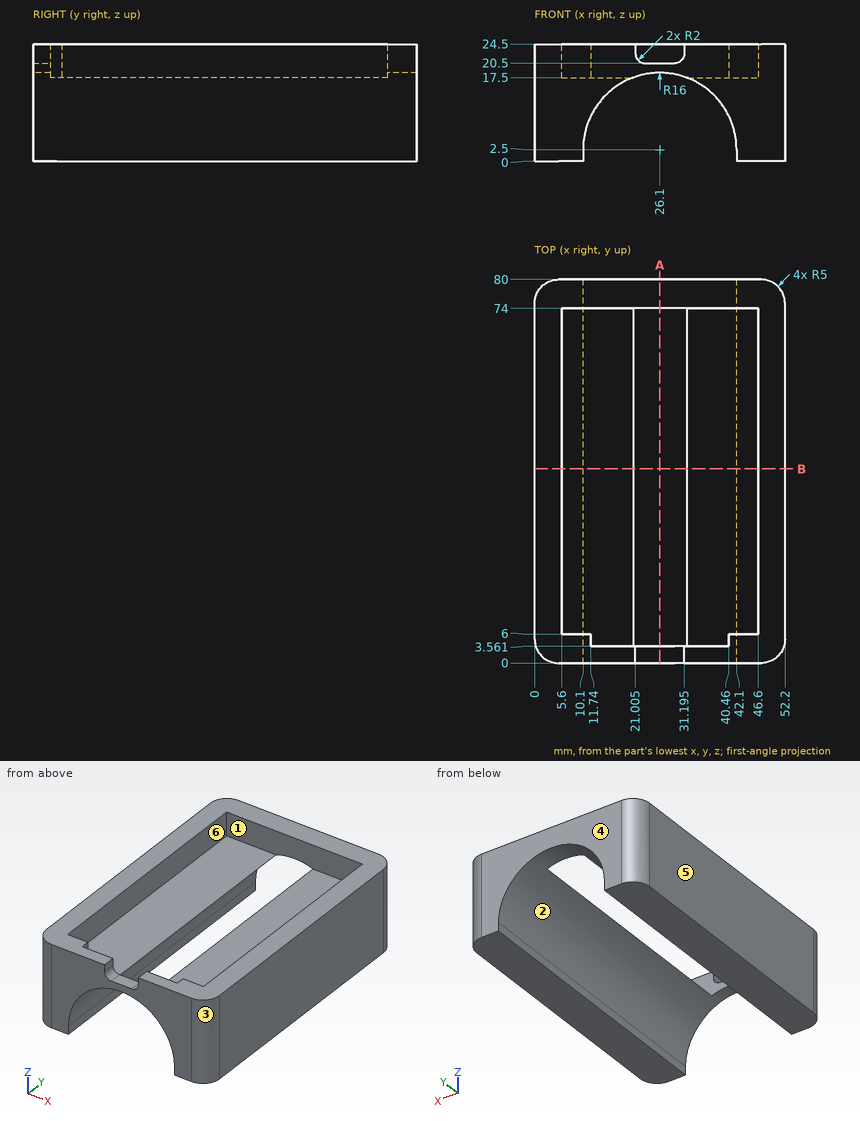
Check sheet for the drawn part. Datum: minimum x, y, z corner. Units: mm. A direction names the side the tool comes from. Round coordinates to 2 decimals unless told otherwise and drop trailing zeros. Order: outer loops, then holes, each group sorted by start corner. A loop starts at its lowest first (then second) coordinate and runs counter-clockwise, first axis right, second up.
(1) Go/stop test with flat-tipped pins: P1, Ø6, axis at x = 29, y = 61.5, coming from the +Z side; P2, Ø1.1, axis at x = 25, y = 2, coming from the +Z side; P3, Ø2, axis at y = 2.5, z = 23, coming from the -X side. Record where each tip stops, or that it passes through.
(2) Draft check along Y on the marked faces 3, 4, 5 and 6. Enter one of: pulls with the +Y half, pulls with the -Y half, needs draft (parallel to the pull), parting line crosses it, or undercut.
(3) Cross-section at A-A, the plane x = 26.1. Enter the section's corners in (y, z).
(4) Access from +Z, -Z, +X, -X, +Y, -Y to the whole of each face (thin tool, end or side, straight path). Record for the marked faces 1 and 2.
(5) Cross-section at B-B, the plane y = 40.5. Enter the section's corners in (x, z).
(6) Scan lines: probe 1 along Y at (x, z) = (45.5, 21.75); probe 2 along X at (y, z) = (50.5, 22.25); probe 3 along Y at (x, z) = (29, 18.75). Record each from-to range of solid material in increasing order.
Check sheet entries:
1. P1: stops at z = 17.5
1. P2: stops at z = 20.5
1. P3: stops at x = 0.23
2. face 3: pulls with the -Y half
2. face 4: pulls with the +Y half
2. face 5: needs draft
2. face 6: undercut
3. outline: (0, 18.5) - (3.56, 18.5) - (3.56, 20.5) - (0, 20.5) - close; (74, 18.5) - (80, 18.5) - (80, 24.5) - (74, 24.5) - close
4. face 1: +Z
4. face 2: -Z, +Y, -Y
5. outline: (0, 0) - (10.1, 0) - (10.1, 2.5) arc R16 cw to (20.53, 17.5) - (5.6, 17.5) - (5.6, 24.5) - (0, 24.5) - close; (31.67, 17.5) arc R16 cw to (42.1, 2.5) - (42.1, 0) - (52.2, 0) - (52.2, 24.5) - (46.6, 24.5) - (46.6, 17.5) - close
6. probe 1: y = 0 to 6, 74 to 80
6. probe 2: x = 0 to 5.6, 46.6 to 52.2
6. probe 3: y = 0 to 3.56, 74 to 80
